```python
from build123d import *

# Parameters (mm, degrees)
SKETCH2_R                   = 3.6195
BEARING_MOUNT_DEPTH         = 6.35
SKETCH3_R                   = 8.0645
BEARING_HOLE_DEPTH          = 4.445
FILLET1_R                   = 6.35
FILLET2_R                   = 0.508
CHAMFER1_SIZE               = 0.508
SKETCH4_W                   = 5.652455718
SKETCH4_H                   = 28.448
MOTOR_MOUNT_DEPTH           = 38.1
FILLET3_R                   = 3.81
MOTOR_MOUNT_STIFFENER_DEPTH = 5.652455718
SKETCH6_R                   = 1.5875
MOTOR_PLATE_HOLES_DEPTH     = 102.044029057
FILLET4_R                   = 0.635
SKETCH7_R                   = 1.5875
MOUNT_HOLES_DEPTH           = 123.601249713
FILLET5_R                   = 2.54


with BuildPart() as part:
    # Sketch2 → Bearing_Mount (new, symmetric)
    with BuildSketch(Plane(origin=(0, 0, 0), x_dir=(0, 0, -1), z_dir=(1, 0, 0))):
        with BuildLine():
            Line((-19.05, 0), (-112.517680526, 0))
            Line((-112.517680526, 0), (-112.517680526, 3.1115))
            Line((-112.517680526, 3.1115), (-68.067680526, 3.1115))
            Line((-68.067680526, 3.1115), (-59.598818102, 17.78))
            ThreePointArc((-59.598818102, 17.78), (-50.8, 22.86), (-42.001181898, 17.78))
            Line((-42.001181898, 17.78), (-33.532319474, 3.1115))
            Line((-33.532319474, 3.1115), (-19.05, 3.1115))
            Line((-19.05, 3.1115), (-19.05, 0))
        make_face()
        with Locations((-50.8, 12.7)):
            Circle(SKETCH2_R, mode=Mode.SUBTRACT)
    extrude(amount=BEARING_MOUNT_DEPTH, both=True)

    # Sketch3 → Bearing_Hole (cut)
    with BuildSketch(Plane(origin=(6.35, 0, 0), x_dir=(0, 0, -1), z_dir=(1, 0, 0))):
        with Locations((-50.8, 12.7)):
            Circle(SKETCH3_R)
    bearing_hole = extrude(amount=-BEARING_HOLE_DEPTH, mode=Mode.SUBTRACT)

    # Mirror1: Bearing_Hole across plane
    add(bearing_hole.mirror(Plane(origin=(0, 0, 0), x_dir=(0, 0, 1), z_dir=(1, 0, 0))), mode=Mode.SUBTRACT)

    # Fillet1
    fillet1_edges = [part.edges().sort_by_distance(p)[0] for p in [
        (0, 3.1115, 68.067680526),
    ]]
    fillet(fillet1_edges, radius=FILLET1_R)

    # Fillet2
    fillet2_edges = [part.edges().sort_by_distance(p)[0] for p in [
        (1.905, 12.7, 58.8645),
        (-1.905, 12.7, 58.8645),
    ]]
    fillet(fillet2_edges, radius=FILLET2_R)

    # Chamfer1
    chamfer1_edges = [part.edges().sort_by_distance(p)[0] for p in [
        (1.905, 12.7, 54.4195),
        (6.35, 12.7, 58.8645),
        (-6.35, 12.7, 58.8645),
        (-1.905, 12.7, 54.4195),
    ]]
    chamfer(chamfer1_edges, length=CHAMFER1_SIZE)

    # Sketch4 → Motor_Mount (add)
    with BuildSketch(Plane(origin=(6.35, 0, 0), x_dir=(0, 0, -1), z_dir=(1, 0, 0))):
        with Locations((-109.691452667, -2.54)):
            Rectangle(SKETCH4_W, SKETCH4_H)
    extrude(amount=MOTOR_MOUNT_DEPTH)

    # Fillet3
    fillet3_edges = [part.edges().sort_by_distance(p)[0] for p in [
        (0, 3.1115, 33.532319474),
    ]]
    fillet(fillet3_edges, radius=FILLET3_R)

    # Sketch5 → Motor_Mount_Stiffener (add)
    with BuildSketch(Plane.XY.offset(112.517680526)):
        Polygon((6.35, 11.684), (-6.35, 3.1115), (6.35, 3.1115), align=None)
    extrude(amount=-MOTOR_MOUNT_STIFFENER_DEPTH)

    # Sketch6 → Motor_Plate_Holes (cut, through all)
    with BuildSketch(Plane(origin=(0, 0, 106.865224808), x_dir=(-1, 0, 0), z_dir=(0, 0, -1))):
        with Locations((-40.894, 7.62)):
            Circle(SKETCH6_R)
        with Locations((-25.908, 7.62)):
            Circle(SKETCH6_R)
        with Locations((-40.894, -12.7)):
            Circle(SKETCH6_R)
        with Locations((-25.908, -12.7)):
            Circle(SKETCH6_R)
    extrude(amount=-MOTOR_PLATE_HOLES_DEPTH, mode=Mode.SUBTRACT)

    # Fillet4
    fillet4_edges = [part.edges().sort_by_distance(p)[0] for p in [
        (6.35, 0, 109.691452667),
    ]]
    fillet(fillet4_edges, radius=FILLET4_R)

    # Sketch7 → Mount-Holes (cut, through all)
    with BuildSketch(Plane(origin=(0, 3.1115, 0), x_dir=(1, 0, 0), z_dir=(0, 1, 0))):
        with Locations(Location((0, -25.4, 0), (0, 0, 270))):
            Circle(SKETCH7_R)
        with Locations(Location((0, -76.2, 0), (0, 0, 270))):
            Circle(SKETCH7_R)
        with Locations(Location((0, -85.09, 0), (0, 0, 270))):
            Circle(SKETCH7_R)
        with Locations(Location((0, -93.98, 0), (0, 0, 270))):
            Circle(SKETCH7_R)
    extrude(amount=-MOUNT_HOLES_DEPTH, mode=Mode.SUBTRACT)

    # Fillet5
    fillet5_edges = [part.edges().sort_by_distance(p)[0] for p in [
        (0, 3.1115, 106.865224808),
    ]]
    fillet(fillet5_edges, radius=FILLET5_R)


solid = part.part
```
CAD build for the part. Positions are in the model's coordinates, mm. A direction names the side the tool comes from. Round coordinates to 2 decimals unless told otherwise and drop trailing zeros. Order: outer loops, then holes, each group sorted by start corner. A loop starts at its lowest first (then second) coordinate and runs counter-clockwise, first axis right, second up. Notation, with made-up numbers: (81, 22.25) - (124, 22.25) arc R31 cw to (124, 49.25) - close; hole circle Ø5 at (-30, 57.25). An arc over 180 degrees is marked (long way). Answer in a Markdown table with one row per item. Add a question column.
(1) Drop flat-ended pins along their axis: pin 1 Ø1.7 at (y, z) = (-12, 109) entering from -X; pin 2 Ø13 at (y, z) = (12.7, 50.8) entering from -X (3 decimals); pin 3 Ø3.5 at (x, y) = (40.894, -12.7) entering from -Z. Give the stop position or say it passes through.
(2) Mould opens along Y. For faces 4 (the face through (-1.905, 9, 48)), 5 (the face through (6.35, 6, 60)), 6 (the face through (0.09, 11.49, 38.37)) say: +Y half, -Y half, draft (parallel to the pull), parting line (faces both ways), or undercut.
(3) 3-axis set-ups, long thin cutter, end or side, ignore diameter. For faces 1 (the face through (0.09, 7.46, 109.39)), 2 (the face through (-6.35, 5, 59)), 3 (the face through (-0.09, 3.94, 68.6)): which of +Z, -Z, +X, -X, +Y, -Y reach the whole face in a straight line?
(4) Band-saw the part on A-A on z = 93.98. List the corners of the cut face in (x, y), and give its area (3 significant figures).
(5) Probe L1, parallel to X at y = 1, z = 85; L2, parallel to Z at x = 14, y = -13.5; L3, parallel to Y at x = 4.5, z = 24.5. List the from-to ranges inside material, lowest first. Write a range as [from, to].
(6) Band-saw the part on B-B on x = 0. Count the separate pieces of the cut face and the enclosed holes in it, and give its area (3 significant figures).
Data:
| question | item | result |
|---|---|---|
| 1 | pin 1 | stops at x = 6.35 |
| 1 | pin 2 | stops at x = -1.905 |
| 1 | pin 3 | stops at z = 106.87 |
| 2 | face 4 | undercut |
| 2 | face 5 | draft |
| 2 | face 6 | +Y half |
| 3 | face 1 | +Z, -X, +Y |
| 3 | face 2 | +Z, -Z, -X, +Y, -Y |
| 3 | face 3 | +X, -X, +Y |
| 4 | outline | (-6.35, 0) - (-1.59, 0) - (-1.59, 3.11) - (-6.35, 3.11) - close; (1.59, 0) - (6.35, 0) - (6.35, 3.11) - (1.59, 3.11) - close |
| 4 | area | 29.6 mm^2 |
| 5 | L1 | x = [-6.35, -1.58], [1.58, 6.35] |
| 5 | L2 | z = [106.87, 112.52] |
| 5 | L3 | y = [0, 3.11] |
| 6 | separate pieces | 5 |
| 6 | enclosed holes | 1 |
| 6 | area | 684 mm^2 |
